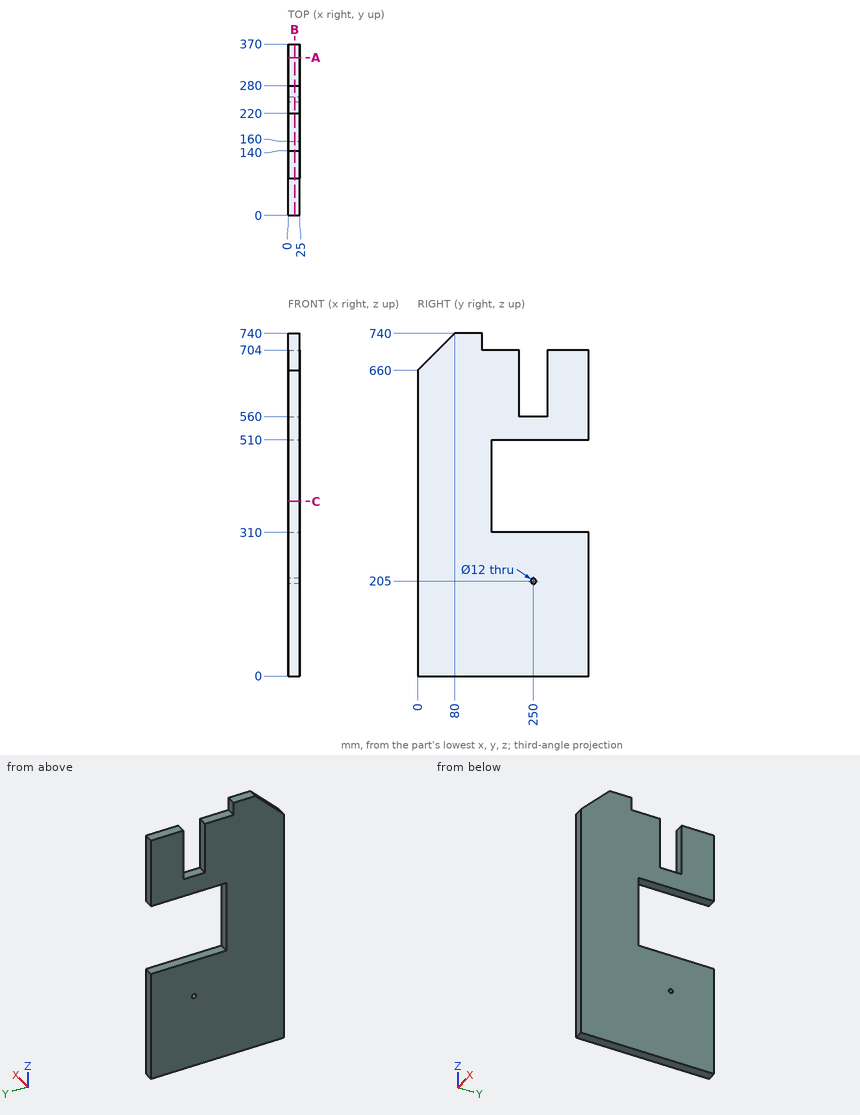
Design review of the part shown in the three views and the two pictorial views. Dimensions are in mm from the part's minimum x, y and z. Round coordinates to 2 decimals unless told otherwise and drop trailing zeros. Order: outer loops, then holes, each group sorted by start corner. A loop starts at its lowest first (then second) coordinate and runs counter-clockwise, first axis right, second up. Notation, with made-up numbers: M -8.75,3 L 34.25,3 A29 cw 34.25,26 Z; hole C 71.5,2.5 d6. An arc over 180 degrees is marked long. Put each result on its own line as item: value.
Q1. Consider section A-A (y = 340.5). State the section outline as (x, z) points.
Reported:
outline: M 0,0 L 25,0 L 25,310 L 0,310 Z; M 0,510 L 25,510 L 25,704 L 0,704 Z
Q2. Consider section C-C (z = 377). State the section outline as (x, y) points.
Reported:
outline: M 0,0 L 25,0 L 25,160 L 0,160 Z
Q3. To check wall thickness, follow line 1 (Z direction, x = 8.25, y = 250); line 2 (Z direction, x = 1.75, y = 211); line 3 (Z direction, x = 9, y = 255). State the ranges of each line that lie inside material, in increasing order.
Reported:
line 1: 0 to 199, 211 to 310, 510 to 560
line 2: 0 to 310, 510 to 704
line 3: 0 to 201.68, 208.32 to 310, 510 to 560
Q4. Insertion check: pin 1 Ø7.5 at (x, y) = (18.5, 295) entering from -Z; pin 2 Ø7.5 at (x, y) = (18.5, 174.5) entering from +Z; pin 3 Ø7.5 at (x, z) = (7.5, 386) entering from +Y; pin 4 Ø7.5 at (x, z) = (11, 718) entering from +Y. Each pin has a flat end and moves straight along its axis. Give the tip position at first contact, or say it passes through.
Reported:
pin 1: z = 0
pin 2: z = 704
pin 3: y = 160
pin 4: y = 140
Q5. Consider section B-B (x = 14.25). State the section outline as (y, z) points.
Reported:
outline: M 0,0 L 370,0 L 370,310 L 160,310 L 160,510 L 370,510 L 370,704 L 280,704 L 280,560 L 220,560 L 220,704 L 140,704 L 140,740 L 80,740 L 0,660 Z; hole C 250,205 d12
